Autodesk Inventor part; units mm, degrees
ref_plane "YZ Plane" through (0, 0, 0) normal (1, 0, 0) x (0, 1, 0)
ref_plane "XZ Plane" through (0, 0, 0) normal (0, 1, 0) x (-1, 0, 0)
ref_plane "XY Plane" through (0, 0, 0) normal (0, 0, 1) x (1, 0, 0)
sketch "Sketch1" plane through (0, 0, 0) normal (0, 1, 0) x (-1, 0, 0)
  line L0 (-10, 22.75) -> (10, 22.75)
  line L1 (10, 22.75) -> (10, -22.75)
  line L2 (10, -22.75) -> (-10, -22.75)
  line L3 (-10, -22.75) -> (-10, 22.75)
  line L4 (-10, 22.75) -> (10, -22.75) construction
  line L5 (10, 22.75) -> (-10, -22.75) construction
  point P0 (0, 0)
  dimension "d0" = 20
  dimension "d1" = 45.5
extrude "Extrusion1" add sketch "Sketch1" along normal blind 1.6
sketch "Sketch2" plane through (0, 1.6, 0) normal (0, 1, 0) x (1, 0, 0)
  line L0 (0, 0) -> (0, 21) construction
  line L1 (0, 21) -> (0, 13) construction
  circle A0 centre (0, 13) radius 8
  line L2 (0, 0) -> (0, -13) construction
  circle A1 centre (0, -13) radius 8
  dimension "d4" = 21
  dimension "d5" = 8
  dimension "d6" = 16
  dimension "d7" = 13
  dimension "d8" = 16
extrude "Extrusion2" add sketch "Sketch2" along normal blind 12
properties part number "Sonar"
Check sheet for the modelled part. Datum: model origin and axes. Units: mm. A direction names the side the tool comes from. Coordinates: 2 decimals unless noted, no trailing zeros. Loops run counter-clockwise (first coordinate to the right, second up) from the corner with the lowest first, then second, coordinate; pieces in that order, holes last.
1) Release check for a two-part mould opening along Z. For faces 1 (the face through (0, 1, -22.75)), 2 (the face through (0, 13.6, 13)), 3 (the face through (0, 1.6, 0)) record: released by +Z, released by -Z, zero draft, split by the parting line, or undercut.
2) Gauge pin test, flat ends, axial feed: pin 1 (4 mm diameter, centred on x = 7.5, z = 7.5, fed in from +Y); pin 2 (3 mm diameter, centred on y = 10, z = -15.5, fed in from -X); pin 3 (2 mm diameter, centred on x = 6.5, y = 12, fed in from -Z); pin 4 (1 mm diameter, centred on x = 2, y = 5, fed in from +Z). Record the tip position at first contact, or that the pin passes through.
3) Sectioned sample at D-D (x = -3.5). Record the boundary of the cut face in (y, z), and give its area (3 significant figures).
4) Access from +Z, -Z, +X, -X, +Y, -Y to the whole of each face (thin tool, end or side, straight path). Record for faces 4 (the face through (-10, 1, 0)), 5 (the face through (-1.73, 7.52, 5.19)).
5) Sectioned sample at C-C (y = 7.75). Record the boundary of the cut face in (x, z), and give its area (3 significant figures).
6) Material ranges on probe 1 along Y at (x, z) = (8.5, 1.5); probe 2 along Z at (x, y) = (6.25, 12); probe 3 along Z at (x, y) = (1, 4.5), recorded low to high.
7) Sectioned sample at A-A (z = 13). Record the boundary of the cut face in (x, y).
8) Sectioned sample at B-B (x = 0). Record the boundary of the cut face in (y, z).
Check sheet entries:
1. face 1: released by -Z
1. face 2: zero draft
1. face 3: undercut
2. pin 1: stops at y = 13.6
2. pin 2: stops at x = -7.94
2. pin 3: stops at z = -18.81
2. pin 4: stops at z = 20.86
3. outline: (0, -22.75) - (1.6, -22.75) - (1.6, -20.19) - (13.6, -20.19) - (13.6, -5.81) - (1.6, -5.81) - (1.6, 5.81) - (13.6, 5.81) - (13.6, 20.19) - (1.6, 20.19) - (1.6, 22.75) - (0, 22.75) - close
3. area: 418 mm2
4. face 4: +Z, -Z, -X, +Y, -Y
4. face 5: +Y
5. outline: circle Ø16 at (0, -13); circle Ø16 at (0, 13)
5. area: 402 mm2
6. probe 1: y = 0 to 1.6
6. probe 2: z = -17.99 to -8.01, 8.01 to 17.99
6. probe 3: z = -20.94 to -5.06, 5.06 to 20.94
7. outline: (-10, 0) - (10, 0) - (10, 1.6) - (8, 1.6) - (8, 13.6) - (-8, 13.6) - (-8, 1.6) - (-10, 1.6) - close
8. outline: (0, -22.75) - (1.6, -22.75) - (1.6, -21) - (13.6, -21) - (13.6, -5) - (1.6, -5) - (1.6, 5) - (13.6, 5) - (13.6, 21) - (1.6, 21) - (1.6, 22.75) - (0, 22.75) - close
